from build123d import *

# Parameters (mm, degrees)
BOSS_EXTRUDE1_DEPTH     = 16
SKETCH3_W               = 96
SKETCH3_H               = 10.65
BOSS_EXTRUDE2_DEPTH     = 16
CUT_EXTRUDE1_DEPTH      = 13.5
CUT_EXTRUDE1_DEPTH_BACK = 13.5
SKETCH7_W               = 16
SKETCH7_H               = 4
HOLE1_D                 = 8.566
HOLE1_DEPTH             = 13.5
HOLE1_CSINK_D           = 9.728
HOLE1_CSINK_ANGLE       = 90
HOLE2_D                 = 8.566
HOLE2_DEPTH             = 16
HOLE2_CSINK_D           = 9.728
HOLE2_CSINK_ANGLE       = 90
HOLE2_TIP               = 2.472791203


with BuildPart() as part:
    # Sketch1 → Revolve1 (revolve)
    with BuildSketch(Plane.XY, mode=Mode.PRIVATE) as revolve1_sk:
        with BuildLine():
            Line((0, 0), (0, 9.8))
            Line((0, 9.8), (0.2, 10))
            Line((0.2, 10), (1, 10))
            Line((1, 10), (2, 11))
            Line((2, 11), (14.95, 11))
            Line((14.95, 11), (15.865685425, 10.084314575))
            ThreePointArc((15.865685425, 10.084314575), (16.125224104, 9.910896374), (16.43137085, 9.85))
            Line((16.43137085, 9.85), (17.2, 9.85))
            ThreePointArc((17.2, 9.85), (17.765685425, 10.084314575), (18, 10.65))
            Line((18, 10.65), (18, 11))
            Line((18, 11), (20, 11))
            Line((20, 11), (20, 0))
            Line((20, 0), (0, 0))
        make_face()
    revolve(revolve1_sk.sketch.rotate(Axis((20, 0, 0), (-1, 0, 0)), 270), axis=Axis((20, 0, 0), (-1, 0, 0)))

    # Sketch2 → Boss-Extrude1 (add)
    with BuildSketch(Plane(origin=(20, 0, 0), x_dir=(0, 0, -1), z_dir=(1, 0, 0))):
        with BuildLine():
            Line((7.25, 11.551515052), (7.25, 13.1))
            ThreePointArc((7.25, 13.1), (7.132842712, 13.382842712), (6.85, 13.5))
            Line((6.85, 13.5), (-6.85, 13.5))
            ThreePointArc((-6.85, 13.5), (-7.132842712, 13.382842712), (-7.25, 13.1))
            Line((-7.25, 13.1), (-7.25, 11.551515052))
            ThreePointArc((-7.25, 11.551515052), (-7.286144803, 11.408754992), (-7.385869565, 11.30039516))
            ThreePointArc((-7.385869565, 11.30039516), (0, -13.5), (7.385869565, 11.30039516))
            ThreePointArc((7.385869565, 11.30039516), (7.286144803, 11.408754992), (7.25, 11.551515052))
        make_face()
    extrude(amount=BOSS_EXTRUDE1_DEPTH)

    # Sketch3 → Revolve2 (revolve)
    with BuildSketch(Plane.XY, mode=Mode.PRIVATE) as revolve2_sk:
        with Locations((84, 5.325)):
            Rectangle(SKETCH3_W, SKETCH3_H)
    revolve(revolve2_sk.sketch.rotate(Axis((132, 0, 0), (-1, 0, 0)), 270), axis=Axis((132, 0, 0), (-1, 0, 0)))

    # Sketch4 → Boss-Extrude2 (add)
    with BuildSketch(Plane(origin=(132, 0, 0), x_dir=(0, 0, -1), z_dir=(1, 0, 0))):
        with BuildLine():
            Line((7.25, 11.551515052), (7.25, 13.1))
            ThreePointArc((7.25, 13.1), (7.132842712, 13.382842712), (6.85, 13.5))
            Line((6.85, 13.5), (-6.85, 13.5))
            ThreePointArc((-6.85, 13.5), (-7.132842712, 13.382842712), (-7.25, 13.1))
            Line((-7.25, 13.1), (-7.25, 11.551515052))
            ThreePointArc((-7.25, 11.551515052), (-7.286144803, 11.408754992), (-7.385869565, 11.30039516))
            ThreePointArc((-7.385869565, 11.30039516), (0, -13.5), (7.385869565, 11.30039516))
            ThreePointArc((7.385869565, 11.30039516), (7.286144803, 11.408754992), (7.25, 11.551515052))
        make_face()
    extrude(amount=BOSS_EXTRUDE2_DEPTH)

    # Sketch5 → Revolve3 (revolve)
    with BuildSketch(Plane.XY, mode=Mode.PRIVATE) as revolve3_sk:
        with BuildLine():
            Line((148, 0), (148, 11))
            Line((148, 11), (150, 11))
            Line((150, 11), (150, 10.65))
            ThreePointArc((150, 10.65), (150.234314575, 10.084314575), (150.8, 9.85))
            Line((150.8, 9.85), (151.56862915, 9.85))
            ThreePointArc((151.56862915, 9.85), (151.874775896, 9.910896374), (152.134314575, 10.084314575))
            Line((152.134314575, 10.084314575), (153.05, 11))
            Line((153.05, 11), (166, 11))
            Line((166, 11), (167, 10))
            Line((167, 10), (167.8, 10))
            Line((167.8, 10), (168, 9.8))
            Line((168, 9.8), (168, 0))
            Line((168, 0), (148, 0))
        make_face()
    revolve(revolve3_sk.sketch.rotate(Axis((168, 0, 0), (-1, 0, 0)), 270), axis=Axis((168, 0, 0), (-1, 0, 0)))

    # Sketch6 → Cut-Extrude1 (cut, two sides: drawn at the far end of the back side and taken through both)
    with BuildSketch(Plane(origin=(0, 0, 0), x_dir=(1, 0, 0), z_dir=(0, 1, 0)).offset(-CUT_EXTRUDE1_DEPTH_BACK)):
        Polygon((139, 24), (139, 8), (168, 8), (168, -8), (139, -8), (139, -24), (184, -24), (184, 24), align=None)
    extrude(amount=CUT_EXTRUDE1_DEPTH + CUT_EXTRUDE1_DEPTH_BACK, mode=Mode.SUBTRACT)

    # Sketch7 → Cut-Revolve1 (revolve, cut)
    with BuildSketch(Plane(origin=(151, 0, 0), x_dir=(0, 0, -1), z_dir=(1, 0, 0)), mode=Mode.PRIVATE) as cut_revolve1_sk:
        with Locations((0, 2)):
            Rectangle(SKETCH7_W, SKETCH7_H)
    revolve(cut_revolve1_sk.sketch.rotate(Axis((151, 0, -8), (0, 0, 1)), 270), axis=Axis((151, 0, -8), (0, 0, 1)), mode=Mode.SUBTRACT)

    # Hole1
    with Locations(Plane(origin=(0, 13.5, 0), x_dir=(1, 0, 0), z_dir=(0, 1, 0))):
        with Locations((28.2, 0)):
            CounterSinkHole(HOLE1_D / 2, HOLE1_CSINK_D / 2, depth=HOLE1_DEPTH, counter_sink_angle=HOLE1_CSINK_ANGLE)

    # Hole2
    with Locations(Plane(origin=(0, 13.5, 0), x_dir=(1, 0, 0), z_dir=(0, 1, 0))):
        with Locations((139.8, 0)):
            CounterSinkHole(HOLE2_D / 2, HOLE2_CSINK_D / 2, depth=HOLE2_DEPTH, counter_sink_angle=HOLE2_CSINK_ANGLE)
            with Locations((0, 0, -(HOLE2_DEPTH + HOLE2_TIP / 2))):  # 120° drill point
                Cone(0, HOLE2_D / 2, HOLE2_TIP, mode=Mode.SUBTRACT)

    # Sketch12 → Cut-Revolve2 (revolve, cut)
    with BuildSketch(Plane.XY, mode=Mode.PRIVATE) as cut_revolve2_sk:
        Polygon((-4, 0), (-4, 4), (50.3, 4), (50.3, 10), (115.3, 10), (115.3, 0), align=None)
    revolve(cut_revolve2_sk.sketch.rotate(Axis((115.3, 0, 0), (-1, 0, 0)), 270), axis=Axis((115.3, 0, 0), (-1, 0, 0)), mode=Mode.SUBTRACT)


solid = part.part
Build history of the part. All positions in model axes, mm. A direction names the side the tool comes from. Coordinates: 2 decimals unless noted, no trailing zeros. Write each loop counter-clockwise with the first axis right and the second up, starting at its lowest first coordinate (ties: lowest second). Pieces come first, ordered by that corner, then holes. Notation, with made-up numbers: (1.5, 42) -> (36.5, 42) arc R6 ccw to (36.5, 51) -> close; hole circle Ø5 at (-19.75, 23.5). An arc over 180 degrees is marked (long way). Use CSV: the item, a comma, the result in double quotes. Start each with the question number.
Q1. Cut at A-A, the plane x = 28.2. List the corners of the cut face in (y, z).
Q2. Flat gauge pins, fed straight in: pin 1 Ø1.2 at (x, y) = (30, 12) entering from +Z; pin 2 Ø0.5 at (x, y) = (138, 12.5) entering from +Z; pin 3 Ø3 at (y, z) = (2, 11.5) entering from +X. Where does each tip first touch, or does it go through?
Q3. 3-axis set-ups, long thin cutter, end or side, ignore diameter. For faces 1 (the flat face through (20, 10, -5)), 2 (the flat face through (50.3, 0.1, -4.3)), 3 (the cylindrical face through (149, 11, 0)), 4 (the flat face through (142, 13.5, -5)), 5 (the cylindrical face through (151.19, 9.85, 0.13)): which of +Z, -Z, +X, -X, +Y, -Y reach the whole face in a straight line?
Q4. Drill centre lines: probe 1 along X at (y, z) = (-10.5, -5.5); probe 2 along Y at (x, z) = (21, 0); probe 3 along Y at (x, z) = (12.5, 0). Where is each one in solid material? Low to high.
Q5. Cut at B-B, the plane x = 84.5. List the corners of the cut face in (y, z), then the cut area to 3 significant figures.
Q6. Cut at C-C, the plane y = 1.5. State how many separate pieces and enclosed holes the cut face has, then the cut area to 4 significant figures.
Q7. Cut at D-D, the plane x = 46. List the corners of the cut face in (y, z).
Q8. Pull direction X, two halves, no side cores. Call faces 6 (the cylindrical face through (160, -11, 0)), 7 (the flat face through (36, 10.1, -3.9)), 8 (the flat face through (139, 0, 10)): released by +X, released by -X, zero draft, split by the parting line, or undercut.
Checked values:
1,outline,"(0, -4.28) -> (0, -4) arc R4 cw to (0, 4) -> (0, 4.28) -> (12.92, 4.28) -> (13.5, 4.86) -> (13.5, 6.85) arc R0.4 ccw to (13.1, 7.25) -> (11.55, 7.25) arc R0.3 cw to (11.3, 7.39) arc R13.5 ccw (long way) to (11.3, -7.39) arc R0.3 cw to (11.55, -7.25) -> (13.1, -7.25) arc R0.4 ccw to (13.5, -6.85) -> (13.5, -4.86) -> (12.92, -4.28) -> close"
2,pin 1,"stops at z = 7.29"
2,pin 2,"stops at z = 7.25"
2,pin 3,"stops at x = 139"
3,face 1,"-X"
3,face 2,"none"
3,face 3,"+X, +Y"
3,face 4,"+Z, -Z, +X, -X, +Y"
3,face 5,"+Y"
4,probe 1,"x = 20 to 36, 132 to 148"
4,probe 2,"y = -13.5 to -4, 4 to 13.5"
4,probe 3,"y = -11 to -4, 4 to 11"
5,outline,"circle Ø21.3 at (0, 0); hole circle Ø20 at (0, 0)"
5,area,"42.2 mm²"
6,separate pieces,"2"
6,enclosed holes,"1"
6,area,"1,695 mm²"
7,outline,"circle Ø21.3 at (0, 0); hole circle Ø8 at (0, 0)"
8,face 6,"zero draft"
8,face 7,"undercut"
8,face 8,"released by +X"
